Design review of the part shown in the three views and the two pictorial views. Dimensions are in mm from the part's minimum x, y and z. Round coordinates to 2 decimals unless told otherwise and drop trailing zeros. Loops run counter-clockwise (first coordinate to the right, second up) from the corner with the lowest first, then second, coordinate; pieces in that order, holes last. Notation, with made-up numbers: (74, 26.25) -> (84, 26.25) arc R9 cw to (84, 41.25) -> close; hole circle Ø9 at (-20, 48.25). An arc over 180 degrees is marked (long way). Use CSV: the item, a comma, the result in double quotes. Start each with the question number.
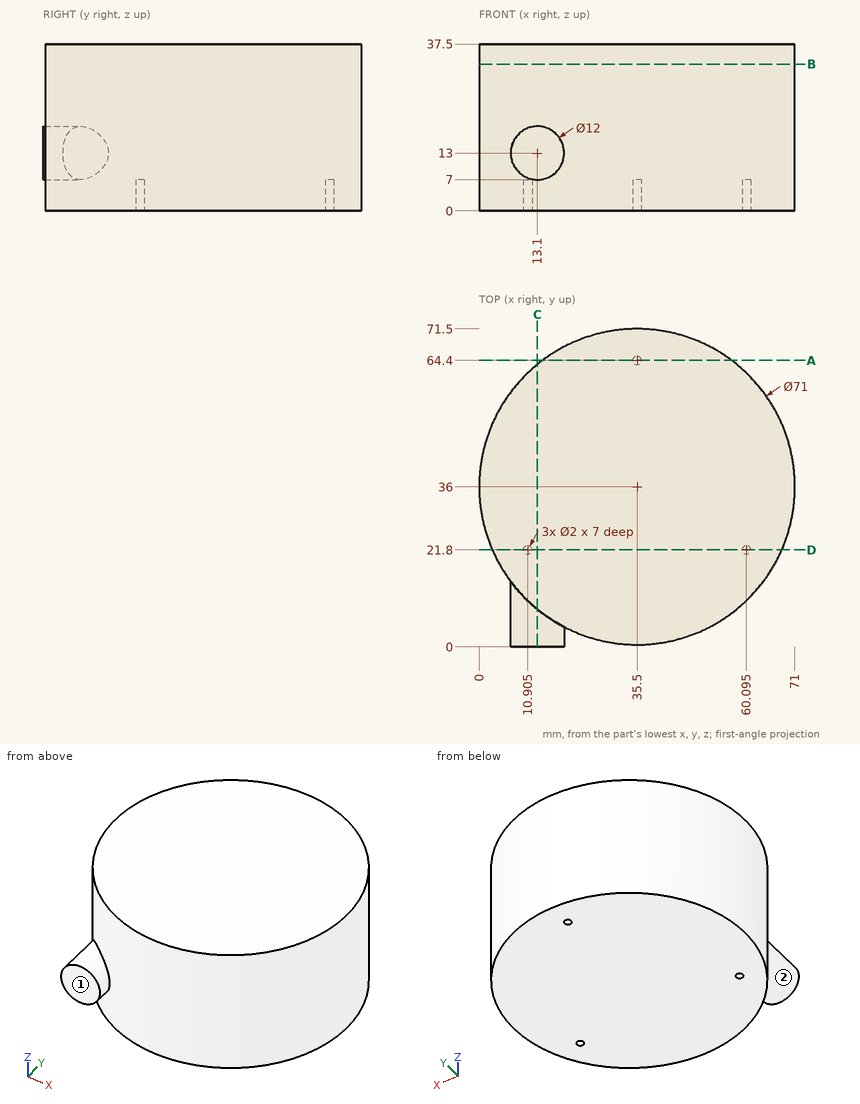
1. Take a section at D-D, the plane y = 21.8. Give the boundary of the cut face in (x, z) (1 decimal).
2. For line 1 along Y through (x, z) = (35.5, 4.5); line 2 along X through (y, z) = (21, 4) (1 decimal); line 3 along X through (y, z) = (36.5, 35.5), list the stretches that pass through material, from the lowest coordinate up. Write a range as from..to.
3. Take a section at B-B, the plane z = 33. Give the boundary of the cut face in (x, y), then the cut area to 3 significant figures.
4. Clearance check with flat-ended pins moving along their axes: P1, Ø1, axis at x = 11, y = 22, coming from the -Z side; P2, Ø8, axis at y = 25.5, z = 10.5, coming from the -X side; P3, Ø1.6, axis at x = 36, y = 65, coming from the -Z side; P4, Ø4, axis at x = 20.5, z = 24.5, coming from the -Y side. State where each tip first meets the part, or that it passes through.
5. Take a section at C-C, the plane x = 13.1. Give the boundary of the cut face in (y, z).
6. The part is to be moulded in two halves that separate along X. For the marked faces 1 and 2, say which applies: pulls with the +X half, pulls with the -X half, needs draft (parallel to the pull), parting line crosses it, or undercut.
7. Take a section at A-A, the plane y = 64.4. Give the boundary of the cut face in (x, z).
Results:
1,outline,"(3, 0) -> (9.9, 0) -> (9.9, 7) -> (11.9, 7) -> (11.9, 0) -> (59.1, 0) -> (59.1, 7) -> (61.1, 7) -> (61.1, 0) -> (68, 0) -> (68, 37.5) -> (3, 37.5) -> close"
2,line 1,"0.5..63.4, 65.4..71.5"
2,line 2,"3.3..10.3, 11.5..59.5, 60.7..67.7"
2,line 3,"0..71"
3,outline,"circle Ø71 at (35.5, 36)"
3,area,"3,960 mm²"
4,P1,"z = 7"
4,P2,"x = 0.6"
4,P3,"z = 0"
4,P4,"y = 2.97"
5,outline,"(0, 7) -> (8.46, 7) -> (8.46, 0) -> (63.54, 0) -> (63.54, 37.5) -> (8.46, 37.5) -> (8.46, 19) -> (0, 19) -> close"
6,face 1,"needs draft"
6,face 2,"undercut"
7,outline,"(14.2, 0) -> (34.5, 0) -> (34.5, 7) -> (36.5, 7) -> (36.5, 0) -> (56.8, 0) -> (56.8, 37.5) -> (14.2, 37.5) -> close"
